CAD build for the part. Positions are in the model's coordinates, mm. A direction names the side the tool comes from. Give positions to 0.01 mm unless a question says otherwise; leave off trailing zeros. Loops run counter-clockwise (first coordinate to the right, second up) from the corner with the lowest first, then second, coordinate; pieces in that order, holes last. Notation, with made-up numbers: (10, -33) - (26, -33) arc R18 cw to (26, -2) - close; hole circle Ø1 at (49, -0.75). An arc over 180 degrees is marked (long way). Return JSON: item names as keys, results as strings.
from build123d import *

# Parameters (mm, degrees)
F0_W      = 10
F0_H      = 25
F1_DEPTH  = 5
F0_R      = 5
F1_FACE_W = 10
F1_FACE_H = 25
F2_DEPTH  = 20
F3_R      = 5
F4_DEPTH  = 68.9


with BuildPart() as f1:
    # F0 (on Front) → F1 (new body)
    with BuildSketch(Plane.XZ):
        with Locations((-15, -7.5)):
            Rectangle(F0_W, F0_H)
    extrude(amount=F1_DEPTH)

    # F0 (on Front) + F1_face (on face) → F2 (join)
    with BuildSketch(Plane.XZ):
        Polygon((10, -20), (10, 20), (-10, 20), (-10, 5), (-10, -20), align=None)
        with Locations((0, -10)):
            Circle(F0_R, mode=Mode.SUBTRACT)
        with Locations((-15, -7.5)):
            Rectangle(F0_W, F0_H)
    with BuildSketch(Plane(origin=(-15, -5, -7.5), x_dir=(1, 0, 0), z_dir=(0, -1, 0))):
        Rectangle(F1_FACE_W, F1_FACE_H)
    extrude(amount=F2_DEPTH)

    # F3 (on Front) → F4 (cut)
    with BuildSketch(Plane.XZ):
        with Locations((0, 10)):
            Circle(F3_R)
    extrude(amount=F4_DEPTH, mode=Mode.SUBTRACT)


solid = f1.part
1. Cut at D-D, the plane z = 3.5. Write the cut outline in (x, y), plus the area to 3 significant figures.
Values follow:
{"outline": "(-20, -25) - (-10, -25) - (-10, -20) - (10, -20) - (10, 0) - (-20, 0) - close", "area": "650 mm²"}
2. Drill centre lines: probe 1 along Z at (x, y) = (0, -14.75); probe 2 along Z at (x, y) = (-2.5, -17.5); probe 3 along Z at (x, y) = (-15.5, -9). Where is each one in solid material? Low to high.
Values follow:
{"probe 1": "z = -20 to -15, -5 to 5, 15 to 20", "probe 2": "z = -20 to -14.33, -5.67 to 5.67, 14.33 to 20", "probe 3": "z = -20 to 5"}
3. Pull direction Z, two halves, no side cores. Call faces 1 (the face through (-20, -12, -8)), 2 (the face through (-0.651, -9.86, 14.957)), 3 (the face through (-15, -12, 5)): +Z half, -Z half, draft (parallel to the pull), parting line (faces both ways), or undercut.
Values follow:
{"face 1": "draft", "face 2": "undercut", "face 3": "+Z half"}
4. Cut at C-C, the plane z = -10. Write the cut outline in (x, y).
Values follow:
{"outline": "(-20, -25) - (-10, -25) - (-10, -20) - (-5, -20) - (-5, 0) - (-20, 0) - close; (5, -20) - (10, -20) - (10, 0) - (5, 0) - close"}
5. Cut at A-A, the plane x = 0. Write the cut outline in (y, z), plus the area to 3 significant figures.
Values follow:
{"outline": "(-20, -20) - (0, -20) - (0, -15) - (-20, -15) - close; (-20, -5) - (0, -5) - (0, 5) - (-20, 5) - close; (-20, 15) - (0, 15) - (0, 20) - (-20, 20) - close", "area": "400 mm²"}
6. Drop flat-ended pins along their axis: P1, Ø10, axis at x = 2, z = -3.5, coming from the -Y side; P2, Ø6, axis at x = 0, z = -10, coming from the -Y side; P3, Ø7.5, axis at y = -10, z = 15, coming from the -X side; P4, Ø4, axis at y = -23, z = -3, coming from the +X side. Give the stop position or say it passes through.
Values follow:
{"P1": "stops at y = -20", "P2": "passes through", "P3": "stops at x = -10", "P4": "stops at x = -10"}
7. Cut at B-B, the plane y = -12.5. Write the cut outline in (x, z).
Values follow:
{"outline": "(-20, -20) - (10, -20) - (10, 20) - (-10, 20) - (-10, 5) - (-20, 5) - close; hole circle Ø10 at (0, -10); hole circle Ø10 at (0, 10)"}
8. Which spindle directions (+Z, -Z, +X, -X, +Y, -Y) get a long thin tool onto all of the face, cutting with end or side? Do faces 4 (the face through (-10, -10, 13)), 5 (the face through (-5, -10, -20)), 6 (the face through (-10, -22, -8)). Say none if no direction does.
Values follow:
{"face 4": "+Z, -X, +Y, -Y", "face 5": "-Z, +X, -X, +Y, -Y", "face 6": "+Z, -Z, +X, -Y"}
